For this review, take the finished solid that the model builds, in its own axes (mm). A direction names the side the tool comes from. Give positions to 0.01 mm unless a question says otherwise; leave off trailing zeros. Loops run counter-clockwise (first coordinate to the right, second up) from the corner with the lowest first, then second, coordinate; pieces in that order, holes last.
```python
from build123d import *

# Parameters (mm, degrees)
SECSKE_W      = 0.508
SECSKE_H      = 2.54
EXTCUT_DEPTH  = 8.112566942
EXTCUTS_COUNT = 14


with BuildPart() as part:
    # SecSke → Body (revolve)
    with BuildSketch(Plane.XY, mode=Mode.PRIVATE) as body_sk:
        with Locations((-0.254, 3.7465)):
            Rectangle(SECSKE_W, SECSKE_H)
    revolve(body_sk.sketch.rotate(Axis((-34.925, 0, 0), (1, 0, 0)), 90), axis=Axis((-34.925, 0, 0), (1, 0, 0)))

    # ExtCutSke → ExtCut (cut, through all)
    with BuildSketch(Plane(origin=(0, 0, 0), x_dir=(0, 0, -1), z_dir=(1, 0, 0))):
        with BuildLine():
            Line((-0.882309718, 5.192903063), (-0.25202333, 3.738013709))
            ThreePointArc((-0.25202333, 3.738013709), (0, 3.7465), (0.25202333, 3.738013709))
            Line((0.25202333, 3.738013709), (0.882309718, 5.192903063))
            ThreePointArc((0.882309718, 5.192903063), (0, 5.267325), (-0.882309718, 5.192903063))
        make_face()
    extcut = extrude(amount=-EXTCUT_DEPTH, mode=Mode.SUBTRACT)

    # ExtCuts: ExtCut ×14 about axis
    extcuts_axis = Axis((0, 0, 0), (1, 0, 0))
    for i in range(1, EXTCUTS_COUNT):
        add(extcut.rotate(extcuts_axis, i * 360 / EXTCUTS_COUNT), mode=Mode.SUBTRACT)


solid = part.part
```
Item 1: Take a section at B-B on z = 0. Give the boundary of the cut face in (x, y).
Answer:
outline: (-0.51, -3.75) - (0, -3.75) - (0, -2.48) - (-0.51, -2.48) - close; (-0.51, 2.48) - (0, 2.48) - (0, 3.75) - (-0.51, 3.75) - close
Item 2: Tool access review of faces 1 (the flat face through (-0.25, 3.7, 2.36)), 2 (the flat face through (-0.25, -3.7, -2.36)), 3 (the flat face through (-0.508, 2, -2)): name each direction out of +Z, -Z, +X, -X, +Y, -Y from which nothing blocks a thin tool from reaching the whole face with its end or side.
Answer:
face 1: +X, -X, +Y
face 2: +X, -X, -Y
face 3: +Z, -Z, -X, +Y, -Y
Item 3: Take a section at C-C on y = 2.75. Give the boundary of the cut face in (x, z), and give its area (3 significant figures).
Answer:
outline: (-0.51, -2.88) - (0, -2.88) - (0, 2.88) - (-0.51, 2.88) - close
area: 2.93 mm2
Item 4: The part is to be moulded in two halves that separate along Z. For faces 4 (the flat face through (0, 2, -2)), 5 (the flat face through (-0.25, 3.686, -2.344)), say which applies: released by +Z, released by -Z, zero draft, split by the parting line, or undercut.
Answer:
face 4: zero draft
face 5: undercut
Item 5: Clearance check with a flat-ended pin moving along its axis: pin 1 Ø4.5 at (y, z) = (0, 0) entering from -X. State where the tip first meets the part, or that it passes through.
Answer:
pin 1: passes through
Item 6: For L1, parallel to Y at x = -0.15, z = -3.25; L2, parallel to Y at x = -0.25, z = 0; L3, parallel to Y at x = -0.2, z = -4.25, list the stretches that pass through material, from the lowest coordinate up.
Answer:
L1: y = -3.82 to -3.44, -2.18 to 2.18, 3.44 to 3.82
L2: y = -3.75 to -2.48, 2.48 to 3.75
L3: y = -2.45 to -1.56, -0.48 to 0.48, 1.56 to 2.45
Item 7: Take a section at A-A on y = 0. Give the boundary of the cut face in (x, z), and give its area (3 significant figures).
Answer:
outline: (-0.51, -5.02) - (0, -5.02) - (0, -2.48) - (-0.51, -2.48) - close; (-0.51, 2.48) - (0, 2.48) - (0, 5.02) - (-0.51, 5.02) - close
area: 2.58 mm2
